Could you check a few things on this model? Use its own coordinates, in mm. Face numbers are marked on the shaded views. A direction names the side the tool comes from. Round coordinates to 2 decimals unless told otherwise and drop trailing zeros. Order: outer loops, then holes, each group sorted by start corner. A loop starts at its lowest first (then second) coordinate and runs counter-clockwise, first axis right, second up. Notation, with made-up numbers: (64, -24) -> (119, -24) arc R21 cw to (119, -19) -> close; hole circle Ø11 at (-24, -38.5). An arc over 180 degrees is marked (long way). Put each result on its own line as item: value. Start each with the question number.
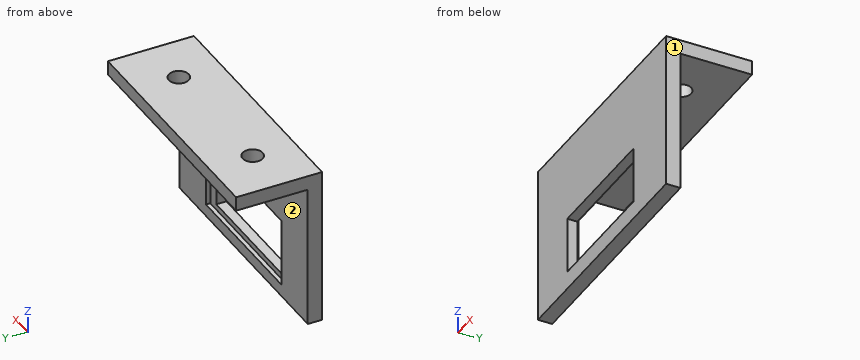
Autodesk Inventor part; units mm, degrees
ref_plane "YZ Plane" through (0, 0, 0) normal (1, 0, 0) x (0, 1, 0)
ref_plane "XZ Plane" through (0, 0, 0) normal (0, 1, 0) x (-1, 0, 0)
ref_plane "XY Plane" through (0, 0, 0) normal (0, 0, 1) x (1, 0, 0)
sketch "Sketch1" plane through (0, 0, 0) normal (0, 1, 0) x (-1, 0, 0)
  line L0 (52.3087, -21.6726) -> (-32.6913, -21.6726)
  line L1 (-32.6913, -21.6726) -> (-32.6913, 38.3274)
  line L2 (-32.6913, 38.3274) -> (52.3087, 38.3274)
  line L3 (52.3087, 38.3274) -> (52.3087, -21.6726)
  dimension "d4" = 60
  dimension "d5" = 85
extrude "Extrusion1" add sketch "Sketch1" along normal blind 20
sketch "Sketch2" plane through (0, 20, 0) normal (0, 1, 0) x (1, 0, 0)
  line L0 (32.6913, 21.6726) -> (-52.3087, 21.6726)
  line L1 (-52.3087, 21.6726) -> (-52.3087, -38.3274)
  line L2 (-52.3087, -38.3274) -> (32.6913, -38.3274)
  line L3 (32.6913, -38.3274) -> (32.6913, 21.6726)
  line L4 (-52.3087, 16.6726) -> (32.6913, 16.6726)
  line L5 (32.6913, 16.6726) -> (32.6913, -33.3274)
  line L6 (32.6913, -33.3274) -> (-52.3087, -33.3274)
  line L7 (-52.3087, -33.3274) -> (-52.3087, 16.6726)
  point P0 (0, 0)
  dimension "d8" = 0
  dimension "d9" = 0
  dimension "d10" = 5
  dimension "d11" = 5
extrude "Extrusion2" cut sketch "Sketch2" against normal blind 15 contours L3 L6 L1 L4
sketch "Sketch3" plane through (0, 5, 0) normal (0, 1, 0) x (1, 0, 0)
  line L0 (-52.3087, 16.6726) -> (32.6913, 16.6726)
  line L1 (-52.3087, -33.3274) -> (-52.3087, 16.6726)
  line L2 (32.6913, -33.3274) -> (-52.3087, -33.3274)
  line L3 (32.6913, 16.6726) -> (32.6913, -33.3274)
  line L4 (-34.8087, 12.4226) -> (15.1913, 12.4226)
  line L5 (15.1913, 12.4226) -> (15.1913, -11.3274)
  line L6 (15.1913, -11.3274) -> (-34.8087, -11.3274)
  line L7 (-34.8087, -11.3274) -> (-34.8087, 12.4226)
  point P0 (0, 0)
  dimension "d14" = 17.5
  dimension "d15" = 17.5
  dimension "d16" = 4.25
  dimension "d17" = 22
extrude "Extrusion3" cut sketch "Sketch3" against normal blind 1.5 contours L4 L5 L6 L7
sketch "Sketch4" plane through (0, 3.5, 0) normal (0, 1, 0) x (1, 0, 0)
  line L0 (-34.8087, 12.4226) -> (15.1913, 12.4226)
  line L1 (-34.8087, -11.3274) -> (-34.8087, 12.4226)
  line L2 (15.1913, -11.3274) -> (-34.8087, -11.3274)
  line L3 (15.1913, 12.4226) -> (15.1913, -11.3274)
  line L4 (-32.8087, 10.4226) -> (11.1913, 10.4226)
  line L5 (11.1913, 10.4226) -> (11.1913, -9.3274)
  line L6 (11.1913, -9.3274) -> (-32.8087, -9.3274)
  line L7 (-32.8087, -9.3274) -> (-32.8087, 10.4226)
  point P0 (0, 0)
  dimension "d20" = 2
  dimension "d21" = 2
  dimension "d22" = 2
  dimension "d23" = 4
extrude "Extrusion4" cut sketch "Sketch4" against normal blind 1 contours L4 L5 L6 L7
sketch "Sketch5" plane through (0, 20, 0) normal (0, 1, 0) x (1, 0, 0)
  line L0 (32.6913, -33.3274) -> (-52.3087, -33.3274)
  line L1 (-52.3087, -33.3274) -> (-52.3087, -38.3274)
  line L2 (-52.3087, -38.3274) -> (32.6913, -38.3274)
  line L3 (32.6913, -38.3274) -> (32.6913, -33.3274)
  line L4 (-52.3087, -33.3274) -> (32.6913, -33.3274)
  line L5 (32.6913, -33.3274) -> (32.6913, -38.3274)
  line L6 (32.6913, -38.3274) -> (-52.3087, -38.3274)
  line L7 (-52.3087, -38.3274) -> (-52.3087, -33.3274)
  point P0 (0, 0)
  dimension "d26" = 0
  dimension "d27" = 0
  dimension "d28" = 0
  dimension "d29" = 0
extrude "Extrusion5" add sketch "Sketch5" against normal blind 35
sketch "Sketch6" plane through (0, 20, 0) normal (0, 1, 0) x (1, 0, 0)
  line L0 (-52.3087, 16.6726) -> (32.6913, 16.6726)
  line L1 (32.6913, 16.6726) -> (32.6913, 21.6726)
  line L2 (32.6913, 21.6726) -> (-52.3087, 21.6726)
  line L3 (-52.3087, 21.6726) -> (-52.3087, 16.6726)
  line L4 (-52.3087, 21.6726) -> (32.6913, 21.6726)
  line L5 (32.6913, 21.6726) -> (32.6913, 16.6726)
  line L6 (32.6913, 16.6726) -> (-52.3087, 16.6726)
  line L7 (-52.3087, 16.6726) -> (-52.3087, 21.6726)
  point P0 (0, 0)
  dimension "d32" = 0
  dimension "d33" = 0
  dimension "d34" = 0
  dimension "d35" = 0
extrude "Extrusion6" cut sketch "Sketch6" against normal blind 20
sketch "Sketch8" plane through (0, 20, 0) normal (0, 1, 0) x (1, 0, 0)
  line L0 (32.6913, -33.3274) -> (-52.3087, -33.3274)
  line L1 (-52.3087, -33.3274) -> (-52.3087, -38.3274)
  line L2 (-52.3087, -38.3274) -> (32.6913, -38.3274)
  line L3 (32.6913, -38.3274) -> (32.6913, -33.3274)
  line L4 (-52.3087, -33.3274) -> (32.6913, -33.3274)
  line L5 (32.6913, -33.3274) -> (32.6913, -38.3274)
  line L6 (32.6913, -38.3274) -> (-52.3087, -38.3274)
  line L7 (-52.3087, -38.3274) -> (-52.3087, -33.3274)
  point P0 (0, 0)
  dimension "d41" = 0
  dimension "d42" = 0
  dimension "d43" = 0
  dimension "d44" = 0
extrude "Extrusion7" add sketch "Sketch8" along normal blind 10
sketch "Sketch9" plane through (0, -15, 0) normal (0, -1, 0) x (1, 0, 0)
  line L0 (-52.3087, 33.3274) -> (32.6913, 33.3274)
  line L1 (32.6913, 33.3274) -> (32.6913, 38.3274)
  line L2 (32.6913, 38.3274) -> (-52.3087, 38.3274)
  line L3 (-52.3087, 38.3274) -> (-52.3087, 33.3274)
  line L4 (-52.3087, 38.3274) -> (32.6913, 38.3274)
  line L5 (32.6913, 38.3274) -> (32.6913, 33.3274)
  line L6 (32.6913, 33.3274) -> (-52.3087, 33.3274)
  line L7 (-52.3087, 33.3274) -> (-52.3087, 38.3274)
  point P0 (0, 0)
  dimension "d47" = 0
  dimension "d48" = 0
  dimension "d49" = 0
  dimension "d50" = 0
extrude "Extrusion8" add sketch "Sketch9" along normal blind 10
sketch "Sketch10" plane through (32.6913, 5, 33.3274) normal (0, 0, -1) x (-1, 0, 0)
  line L0 (85, 25) -> (85, 0)
  line L1 (0, 25) -> (85, 25)
  circle A0 centre (18, 9.75) radius 3.5
  circle A1 centre (67, 9.75) radius 3.5
  point P0 (32.6913, -5)
  dimension "d53" = 15.25
  dimension "d55" = 15.25
  dimension "d58" = 7
  dimension "d59" = 7
  dimension "d70" = 49
  dimension "d71" = 18
extrude "Extrusion9" cut sketch "Sketch10" against normal blind 5
sketch "Sketch11" plane through (32.6913, 0, 33.3274) normal (0, 0, -1) x (-1, 0, 0)
  line L0 (0, 0) -> (0, -25)
  line L1 (85, -25) -> (0, -25)
  line L2 (85, 0) -> (85, -25)
  circle A0 centre (18, -9.75) radius 3.5
  circle A1 centre (67, -9.75) radius 3.5
  point P0 (32.6913, 0)
  dimension "d62" = 18
  dimension "d63" = 18
  dimension "d64" = 7
  dimension "d65" = 7
  dimension "d66" = 15.25
  dimension "d67" = 15.25
extrude "Extrusion10" cut sketch "Sketch11" against normal blind 5
sketch "Sketch13" plane through (0, 5, 0) normal (0, 1, 0) x (1, 0, 0)
  line L0 (-52.3087, 16.6726) -> (32.6913, 16.6726)
  line L1 (32.6913, -33.3274) -> (-52.3087, -33.3274)
  line L2 (32.6913, 16.6726) -> (32.6913, -33.3274)
  line L3 (32.6913, 16.6726) -> (29.6913, 16.6726)
  line L4 (29.6913, 16.6726) -> (29.6913, -33.3274)
  line L5 (29.6913, -33.3274) -> (32.6913, -33.3274)
  line L6 (32.6913, -33.3274) -> (32.6913, 16.6726)
  point P0 (0, 0)
  dimension "d72" = 0
  dimension "d73" = 0
  dimension "d74" = 0
  dimension "d75" = 3
extrude "Extrusion11" add sketch "Sketch13" along normal blind 20
sketch "Sketch14" plane through (32.6913, 0, 33.3274) normal (1, 0, 0) x (0, 0, -1)
  line L0 (50, 0) -> (50, 25)
  line L1 (50, 0) -> (0, 0)
  circle A0 centre (41.5, 10) radius 2
  circle A1 centre (27.5, 10) radius 2
  point P0 (33.3274, 0)
  dimension "d78" = 4
  dimension "d79" = 4
  dimension "d80" = 8.5
  dimension "d81" = 10
  dimension "d82" = 22.5
  dimension "d83" = 10
extrude "Extrusion12" cut sketch "Sketch14" against normal blind 5
sketch "Sketch15" plane through (0, -25, 0) normal (0, -1, 0) x (1, 0, 0)
  line L0 (-52.3087, 33.3274) -> (32.6913, 33.3274)
  line L1 (32.6913, 33.3274) -> (32.6913, 38.3274)
  line L2 (32.6913, 38.3274) -> (-52.3087, 38.3274)
  line L3 (-52.3087, 38.3274) -> (-52.3087, 33.3274)
  line L4 (-52.3087, 38.3274) -> (32.6913, 38.3274)
  line L5 (32.6913, 38.3274) -> (32.6913, 33.3274)
  line L6 (32.6913, 33.3274) -> (-52.3087, 33.3274)
  line L7 (-52.3087, 33.3274) -> (-52.3087, 38.3274)
  point P0 (0, 0)
  dimension "d86" = 0
  dimension "d87" = 0
  dimension "d88" = 0
  dimension "d89" = 0
extrude "Extrusion13" cut sketch "Sketch15" against normal blind 25
sketch "Sketch16" plane through (15.1913, 5, -12.4226) normal (-1, 0, 0) x (0, 0, 1)
  line L0 (0, 0) -> (23.75, 0)
  line L1 (0, 0) -> (0, -1.5)
  line L2 (0, -1.5) -> (23.75, -1.5)
  line L3 (23.75, 0) -> (23.75, -1.5)
  point P0 (12.4226, -5)
sketch "Sketch17" plane through (0, 2.5, 0) normal (0, 1, 0) x (1, 0, 0)
  line L0 (-32.8087, 10.4226) -> (11.1913, 10.4226)
  line L1 (-32.8087, -9.3274) -> (-32.8087, 10.4226)
  line L2 (11.1913, -9.3274) -> (-32.8087, -9.3274)
  line L3 (11.1913, 10.4226) -> (11.1913, -9.3274)
  line L4 (-32.8087, 10.4226) -> (11.1913, 10.4226)
  line L5 (11.1913, 10.4226) -> (11.1913, -9.3274)
  line L6 (11.1913, -9.3274) -> (-32.8087, -9.3274)
  line L7 (-32.8087, -9.3274) -> (-32.8087, 10.4226)
  point P0 (0, 0)
  dimension "d93" = 0
  dimension "d94" = 0
  dimension "d95" = 0
  dimension "d96" = 0
extrude "Extrusion14" cut sketch "Sketch17" along normal mid plane 5
sketch "Sketch18" plane through (0, 25, 0) normal (0, 1, 0) x (1, 0, 0)
  line L0 (32.6913, 16.6726) -> (29.6913, 16.6726)
  line L1 (29.6913, 16.6726) -> (29.6913, -33.3274)
  line L2 (32.6913, -33.3274) -> (29.6913, -33.3274)
  line L3 (32.6913, -33.3274) -> (32.6913, 16.6726)
  line L4 (29.6913, 16.6726) -> (32.6913, 16.6726)
  line L5 (32.6913, 16.6726) -> (32.6913, -33.3274)
  line L6 (32.6913, -33.3274) -> (29.6913, -33.3274)
  line L7 (29.6913, -33.3274) -> (29.6913, 16.6726)
  point P0 (0, 0)
  dimension "d99" = 0
  dimension "d100" = 0
  dimension "d101" = 0
  dimension "d102" = 0
extrude "Extrusion15" cut sketch "Sketch18" against normal blind 20
properties part number "sampleholderdraft5"
1. If we section it at D-D, the plane x = -46: Please give me the cut outline in (y, z), then the cut area to 3 significant figures.
2. If we section it at B-B, the plane x = -3.5: Please give me the cut outline in (y, z), then the cut area to 3 significant figures.
3. For pin 1 Ø2 at (x, y) = (-20, 16.5) entering from -Z; pin 2 Ø19 at (x, z) = (-1, 0.5) entering from +Y; pin 3 Ø5.5 at (x, y) = (14.69, 14.75) entering from -Z; pin 4 Ø6 at (x, z) = (13.5, 30) entering from +Y, each with a flat end and sliding along its axis, tell me the tip position at first contact or that it passes through.
4. Which directions (+Z, -Z, +X, -X, +Y, -Y) give clear straight access to the entire face, cutting with the end or side of a thin tool? Please do the marked faces 1 and 2.
5. I need wall thicknesses on L1, parallel to Z at x = 3, y = 15; L2, parallel to Y at x = 4, z = 15.5. Which ranges of each line are inside material? Lowest first, please.
6. If we section it at A-A, the plane y = 14.75: Please give me the cut outline in (x, z).
7. If we section it at C-C, the plane z = -1.5: Please give me the cut outline in (x, y).
Results below:
1. outline: (0, -16.67) -> (5, -16.67) -> (5, 33.33) -> (30, 33.33) -> (30, 38.33) -> (0, 38.33) -> close
1. area: 400 mm2
2. outline: (0, -16.67) -> (5, -16.67) -> (5, -12.42) -> (3.5, -12.42) -> (3.5, -10.42) -> (0, -10.42) -> close; (0, 9.33) -> (3.5, 9.33) -> (3.5, 11.33) -> (5, 11.33) -> (5, 33.33) -> (30, 33.33) -> (30, 38.33) -> (0, 38.33) -> close
2. area: 295 mm2
3. pin 1: z = 33.33
3. pin 2: y = 3.5
3. pin 3: through
3. pin 4: y = 5
4. face 1: +Z, -Z, +X, +Y, -Y
4. face 2: -Z, +X, -X, +Y
5. L1: 33.33 to 38.33
5. L2: 0 to 5
6. outline: (-52.31, 33.33) -> (-37.81, 33.33) -> (-37.81, 38.33) -> (-52.31, 38.33) -> close; (-30.81, 33.33) -> (11.19, 33.33) -> (11.19, 38.33) -> (-30.81, 38.33) -> close; (18.19, 33.33) -> (32.69, 33.33) -> (32.69, 38.33) -> (18.19, 38.33) -> close
7. outline: (-52.31, 0) -> (-32.81, 0) -> (-32.81, 3.5) -> (-34.81, 3.5) -> (-34.81, 5) -> (-52.31, 5) -> close; (11.19, 0) -> (32.69, 0) -> (32.69, 5) -> (15.19, 5) -> (15.19, 3.5) -> (11.19, 3.5) -> close
